Part model, mm, in its own coordinate system. Face numbers are marked on the shaded views. A direction names the side the tool comes from. Give positions to 0.01 mm unless a question says otherwise; leave off trailing zeros. Order: outer loops, then holes, each group sorted by start corner. A loop starts at its lowest first (then second) coordinate and runs counter-clockwise, first axis right, second up. Notation, with made-up numbers: M 53,28 L 107,28 A13 ccw 107,47 Z; hole C -5.5,48.25 d11. An arc over 180 degrees is marked long. Return JSON: item names as keys, results as strings.
from build123d import *

# Parameters (mm, degrees)
BASPROSKE_W             = 5
BASPROSKE_H             = 4.2
TOOTHCUT_DEPTH          = 8.764019578
TEETHCUTS_COUNT         = 10
TEETHCUTS_ANGLE         = 324
BORSKE_R                = 1.5
BORE_DEPTH              = 50.0000508
CROQUIS1_R              = 4.25
CROQUIS1_R_2            = 3.25
SALIENTE_EXTRUIR1_DEPTH = 5
CROQUIS2_R              = 3.25
SALIENTE_EXTRUIR2_DEPTH = 2
SALIENTE_EXTRUIR3_DEPTH = 2


with BuildPart() as part:
    # BasProSke → Base-Revolve (revolve)
    with BuildSketch(Plane(origin=(0, 0, 0), x_dir=(1, 0, 0), z_dir=(0, 1, 0)), mode=Mode.PRIVATE) as base_revolve_sk:
        with Locations((2.5, 2.1)):
            Rectangle(BASPROSKE_W, BASPROSKE_H)
    revolve(base_revolve_sk.sketch.rotate(Axis((-10, 0, 0), (1, 0, 0)), 180), axis=Axis((-10, 0, 0), (1, 0, 0)))

    # TooCutSke → ToothCut (cut, through all)
    with BuildSketch(Plane(origin=(0, 0, 0), x_dir=(0, 0, -1), z_dir=(1, 0, 0))):
        with BuildLine():
            ThreePointArc((0.415506654, 2.590893711), (0, 2.624), (-0.415506654, 2.590893711))
            ThreePointArc((-0.415506654, 2.590893711), (-0.596160737, 3.451685568), (-1.254578949, 4.034852763))
            ThreePointArc((-1.254578949, 4.034852763), (0, 4.2254), (1.254578949, 4.034852763))
            ThreePointArc((1.254578949, 4.034852763), (0.596160737, 3.451685568), (0.415506654, 2.590893711))
        make_face()
    toothcut = extrude(amount=TOOTHCUT_DEPTH, mode=Mode.SUBTRACT)

    # TeethCuts: ToothCut ×10 about axis
    teethcuts_axis = Axis((-10, 0, 0), (1, 0, 0))
    for i in range(1, TEETHCUTS_COUNT):
        add(toothcut.rotate(teethcuts_axis, i * TEETHCUTS_ANGLE / (TEETHCUTS_COUNT - 1)), mode=Mode.SUBTRACT)

    # BorSke → Bore (cut, symmetric)
    with BuildSketch(Plane(origin=(0, 0, 0), x_dir=(0, 0, -1), z_dir=(1, 0, 0))):
        with Locations(Location((0, 0, 0), (0, 0, 180))):
            Circle(BORSKE_R)
    extrude(amount=BORE_DEPTH, both=True, mode=Mode.SUBTRACT)

    # Croquis1 → Saliente-Extruir1 (add)
    with BuildSketch(Plane.ZY):
        Circle(CROQUIS1_R)
        with Locations(Location((0, 0, 0), (0, 0, 189.396976621))):
            Circle(CROQUIS1_R_2, mode=Mode.SUBTRACT)
    extrude(amount=SALIENTE_EXTRUIR1_DEPTH)

    # Croquis2 → Saliente-Extruir2 (add)
    with BuildSketch(Plane.ZY):
        Circle(CROQUIS2_R)
    extrude(amount=SALIENTE_EXTRUIR2_DEPTH)

    # Croquis3 → Saliente-Extruir3 (add)
    with BuildSketch(Plane.ZY.offset(2)):
        with BuildLine():
            Line((-1.95, 2.6), (-1.95, -2.6))
            ThreePointArc((-1.95, -2.6), (-3.25, 0), (-1.95, 2.6))
        make_face()
    extrude(amount=SALIENTE_EXTRUIR3_DEPTH)


solid = part.part
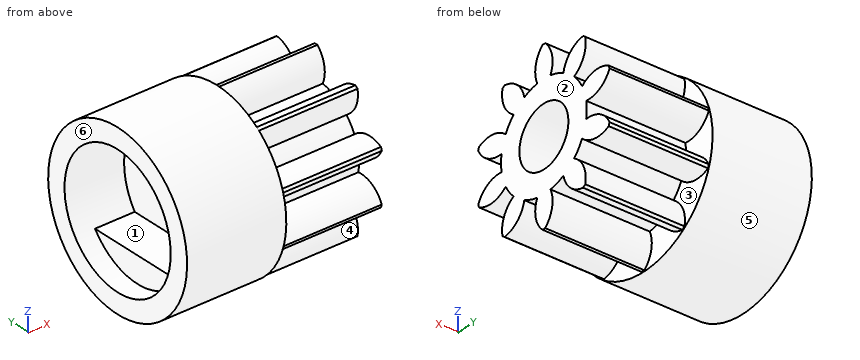
Q1. Band-saw the part on C-C (x = -3). Give the cut face in (y, z), then the cut area to 3 significant figures.
Established:
{"outline": "C 0,0 d8.5; hole M -2.6,-1.95 L 2.6,-1.95 A3.25 ccw long Z", "area": "28.3 mm²"}
Q2. Two-plate mould, pull along Z, no slides. Class the marked faces 4, 5 and 6: +Z half, -Z half, draft (parallel to the pull), parting line (faces both ways), or undercut.
Established:
{"face 4": "undercut", "face 5": "parting line", "face 6": "draft"}
Q3. 3-axis set-ups, long thin cutter, end or side, ignore diameter. For the marked faces 1, 2 and 3: which of +Z, -Z, +X, -X, +Y, -Y reach the whole face in a straight line?
Established:
{"face 1": "-X", "face 2": "+Z, -Z, +X, +Y, -Y", "face 3": "+X"}
Q4. Probe line 1 along Y through (x, z) = (-4.3, 0); line 2 along Y through (x, z) = (2.35, 0); line 3 along X through (y, z) = (3.25, -2.25). List the from-to ranges inside material, lowest first.
Established:
{"line 1": "y = -4.25 to -3.25, 3.25 to 4.25", "line 2": "y = -2.62 to -1.5, 1.5 to 2.62", "line 3": "x = -5 to 0"}
Q5. Band-saw the part on B-B (y = 1). Give the cut face in (x, z), then the cut area to 3 significant figures.
Established:
{"outline": "M -5,-4.13 L 0,-4.13 L 0,-2.43 L 5,-2.43 L 5,-1.12 L 0,-1.12 L 0,1.12 L 5,1.12 L 5,2.43 L 0,2.43 L 0,4.13 L -5,4.13 L -5,3.09 L -2,3.09 L -2,-1.95 L -4,-1.95 L -4,-3.09 L -5,-3.09 Z", "area": "38.1 mm²"}
Q6. Band-saw the part on D-D (y = -0.25). Give the cut face in (x, z), then the cut area to 3 significant figures.
Established:
{"outline": "M -5,-4.24 L 0,-4.24 L 0,-4.01 L 5,-4.01 L 5,-1.48 L 0,-1.48 L 0,1.48 L 5,1.48 L 5,4.01 L 0,4.01 L 0,4.24 L -5,4.24 L -5,3.24 L -2,3.24 L -2,-1.95 L -4,-1.95 L -4,-3.24 L -5,-3.24 Z", "area": "50.9 mm²"}
Q7. Band-saw the part on A-A (z = 0.75). Give the cut face in (x, y).
Established:
{"outline": "M -5,-4.18 L 0,-4.18 L 0,-3.67 L 5,-3.67 L 5,-1.3 L 0,-1.3 L 0,1.3 L 5,1.3 L 5,3.67 L 0,3.67 L 0,4.18 L -5,4.18 L -5,3.16 L -2,3.16 L -2,-3.16 L -5,-3.16 Z"}
Q8. Pin check, flat tips, straight feed: pin 1 (2 mm diameter, centred on y = 2.5, z = 0.5, fed in from -X); pin 2 (1 mm diameter, centred on x = -3.5, z = -3.5, fed in from -Y); pin 3 (1 mm diameter, centred on y = -1, z = -2.5, fed in from -X); pin 4 (2 mm diameter, centred on x = -2, z = 2.5, fed in from -Y). Stop position of each tip, or through.
Established:
{"pin 1": "stops at x = -5", "pin 2": "stops at y = -3.01", "pin 3": "stops at x = -4", "pin 4": "stops at y = -3.98"}
